For this review, take the finished solid that the model builds, in its own axes (mm). A direction names the side the tool comes from. Give positions to 0.01 mm unless a question says otherwise; leave off trailing zeros. Write each loop counter-clockwise with the first axis right and the second up, starting at its lowest first coordinate (ties: lowest second). Pieces come first, ordered by that corner, then holes. Notation, with made-up numbers: (30, -33) -> (52, -33) arc R8 cw to (52, -28) -> close; hole circle Ø6 at (40.5, 43.5). An arc over 180 degrees is marked (long way). Return JSON: item names as keys, results as strings.
from build123d import *

# Parameters (mm, degrees)
BOSS_EXTRUDE1_DEPTH  = 19.05
CUT_EXTRUDE1_DEPTH   = 23.803574111
SKETCH2_4_W          = 12.954
SKETCH2_4_H          = 1.7018
CUT_EXTRUDE2_DEPTH   = 18.25625
SKETCH6_W            = 0.608326788
SKETCH6_H            = 1.5875
SKETCH8_W            = 2.576826788
SKETCH8_H            = 1.5875
SKETCH9_W            = 12.954
SKETCH9_H            = 5.08
SKETCH9_H_2          = 2.159
CUT_EXTRUDE3_DEPTH   = 6.35
BOSS_EXTRUDE2_DEPTH  = 2.54
SKETCH11_W           = 1.905
SKETCH11_H           = 0.127
BOSS_EXTRUDE3_DEPTH  = 0.254
FILLET1_R            = 0.508
FILLET2_R            = 0.0635
BOSS_EXTRUDE4_DEPTH  = 1.27
BOSS_EXTRUDE5_DEPTH  = 1.905
FILLET1_OF_MIRROR1_R = 0.508


with BuildPart() as part:
    # Sketch1 → Boss-Extrude1 (new body)
    with BuildSketch(Plane(origin=(0, 0, 0), x_dir=(1, 0, 0), z_dir=(0, 1, 0))):
        with BuildLine():
            Line((-0.79375, 9.109483901), (-0.79375, 8.535673212))
            ThreePointArc((-0.79375, 8.535673212), (-7.424002774, 4.28625), (-7.78898484, -3.580428942))
            Line((-7.78898484, -3.580428942), (-8.285919473, -3.867334286))
            ThreePointArc((-8.285919473, -3.867334286), (-7.918936292, -4.572), (-7.492169473, -5.242149615))
            Line((-7.492169473, -5.242149615), (-6.99523484, -4.95524427))
            ThreePointArc((-6.99523484, -4.95524427), (0, -8.5725), (6.99523484, -4.95524427))
            Line((6.99523484, -4.95524427), (7.492169473, -5.242149615))
            ThreePointArc((7.492169473, -5.242149615), (7.918936292, -4.572), (8.285919473, -3.867334286))
            Line((8.285919473, -3.867334286), (7.78898484, -3.580428942))
            ThreePointArc((7.78898484, -3.580428942), (7.424002774, 4.28625), (0.79375, 8.535673212))
            Line((0.79375, 8.535673212), (0.79375, 9.109483901))
            ThreePointArc((0.79375, 9.109483901), (0, 9.144), (-0.79375, 9.109483901))
        make_face()
    extrude(amount=BOSS_EXTRUDE1_DEPTH)

    # Sketch2 → Cut-Extrude1 (cut, through all)
    with BuildSketch(Plane(origin=(0, 19.05, 0), x_dir=(1, 0, 0), z_dir=(0, 1, 0))):
        with BuildLine():
            Line((-4.543615348, 4.303093955), (-3.175, 2.4638))
            Line((-3.175, 2.4638), (3.175, 2.4638))
            Line((3.175, 2.4638), (4.543615348, 4.303093955))
            ThreePointArc((4.543615348, 4.303093955), (4.598203733, 4.928342625), (4.064, 5.2578))
            Line((4.064, 5.2578), (-4.064, 5.2578))
            ThreePointArc((-4.064, 5.2578), (-4.598203733, 4.928342625), (-4.543615348, 4.303093955))
        make_face()
    extrude(amount=-CUT_EXTRUDE1_DEPTH, mode=Mode.SUBTRACT)

    # Sketch2_4 → Cut-Extrude2 (cut)
    with BuildSketch(Plane(origin=(0, 19.05, 0), x_dir=(1, 0, 0), z_dir=(0, 1, 0))):
        with Locations((0, 1.6129)):
            Rectangle(SKETCH2_4_W, SKETCH2_4_H)
    extrude(amount=-CUT_EXTRUDE2_DEPTH, mode=Mode.SUBTRACT)

    # Sketch6 → Cut-Revolve2 (revolve, cut)
    with BuildSketch(Plane(origin=(0, 0, 0), x_dir=(0, 0, -1), z_dir=(1, 0, 0)), mode=Mode.PRIVATE) as cut_revolve2_sk:
        with Locations((8.839836606, 0.79375)):
            Rectangle(SKETCH6_W, SKETCH6_H)
    revolve(cut_revolve2_sk.sketch.rotate(Axis((0, 19.730213777, 0), (0, -1, 0)), 180), axis=Axis((0, 19.730213777, 0), (0, -1, 0)), mode=Mode.SUBTRACT)

    # Sketch8 → Revolve2 (revolve)
    with BuildSketch(Plane(origin=(0, 0, 0), x_dir=(0, 0, -1), z_dir=(1, 0, 0)), mode=Mode.PRIVATE) as revolve2_sk:
        with Locations((9.824086606, 0.79375)):
            Rectangle(SKETCH8_W, SKETCH8_H)
    revolve(revolve2_sk.sketch.rotate(Axis((0, 4.48386458, 0), (0, -1, 0)), 180), axis=Axis((0, 4.48386458, 0), (0, -1, 0)))

    # Sketch9 → Cut-Extrude3 (cut)
    with BuildSketch(Plane(origin=(0, 19.05, 0), x_dir=(1, 0, 0), z_dir=(0, 1, 0))):
        with Locations((0, -1.778)):
            Rectangle(SKETCH9_W, SKETCH9_H)
        with Locations((0, 3.5433)):
            Rectangle(SKETCH9_W, SKETCH9_H_2)
    extrude(amount=-CUT_EXTRUDE3_DEPTH, mode=Mode.SUBTRACT)

    # Sketch10 → Boss-Extrude2 (add)
    with BuildSketch(Plane(origin=(0, 12.7, 0), x_dir=(1, 0, 0), z_dir=(0, 1, 0))):
        Polygon((-3.175, 2.4638), (-4.025504259, 3.6068), (-5.08, 3.6068), (-5.08, 2.4638), align=None)
    boss_extrude2 = extrude(amount=BOSS_EXTRUDE2_DEPTH)

    # Sketch11 → Boss-Extrude3 (add)
    with BuildSketch(Plane.XY.offset(-2.4638)):
        with Locations((-4.1275, 15.1765)):
            Rectangle(SKETCH11_W, SKETCH11_H)
    boss_extrude3 = extrude(amount=BOSS_EXTRUDE3_DEPTH)

    # Fillet1
    fillet1_edges = [part.edges().sort_by_distance(p)[0] for p in [
        (-4.55275213, 12.7, -3.6068),
    ]]
    fillet(fillet1_edges, radius=FILLET1_R)

    # Fillet2
    fillet2_edges = [part.edges().sort_by_distance(p)[0] for p in [
        (-4.1275, 15.113, -2.4638),
    ]]
    fillet(fillet2_edges, radius=FILLET2_R)

    # Sketch12 → Boss-Extrude4 (add)
    with BuildSketch(Plane(origin=(0, 15.24, 0), x_dir=(1, 0, 0), z_dir=(0, 1, 0))):
        Polygon((-3.175, 2.2098), (-3.175, 2.4638), (-4.025504259, 3.6068), (-5.08, 3.6068), (-5.08, 2.2098), align=None)
    boss_extrude4 = extrude(amount=BOSS_EXTRUDE4_DEPTH)

    # Sketch13 → Boss-Extrude5 (add)
    with BuildSketch(Plane(origin=(-3.175, 0, 0), x_dir=(0, 0, -1), z_dir=(1, 0, 0))):
        Polygon((2.2098, 15.113), (1.403241674, 16.51), (2.2098, 16.51), align=None)
    boss_extrude5 = extrude(amount=-BOSS_EXTRUDE5_DEPTH)

    # Mirror1: Boss-Extrude2, Boss-Extrude3, Boss-Extrude4, Boss-Extrude5 across plane
    add(boss_extrude2.mirror(Plane(origin=(0, 0, 0), x_dir=(0, 0, 1), z_dir=(1, 0, 0))))
    add(boss_extrude3.mirror(Plane(origin=(0, 0, 0), x_dir=(0, 0, 1), z_dir=(1, 0, 0))))
    add(boss_extrude4.mirror(Plane(origin=(0, 0, 0), x_dir=(0, 0, 1), z_dir=(1, 0, 0))))
    add(boss_extrude5.mirror(Plane(origin=(0, 0, 0), x_dir=(0, 0, 1), z_dir=(1, 0, 0))))

    # Fillet1 of Mirror1
    fillet1_of_mirror1_edges = [part.edges().sort_by_distance(p)[0] for p in [
        (4.55275213, 12.7, -3.6068),
    ]]
    fillet(fillet1_of_mirror1_edges, radius=FILLET1_OF_MIRROR1_R)


solid = part.part
1. For pin 1 (1.7 mm diameter, centred on x = 5, y = 5, fed in from +Z); pin 2 (3 mm diameter, centred on y = 15, z = -3, fed in from -X); pin 3 (3 mm diameter, centred on x = 1.5, y = 17, fed in from -Z), all flat-tipped, find the tip position at first contact; note any pin that passes through.
Results found:
{"pin 1": "stops at z = 7.5", "pin 2": "stops at x = -8.44", "pin 3": "stops at z = -9.14"}
2. Add section B-B, the plane y = 5.75. State the section outline as (x, z) points (1 decimal).
Results found:
{"outline": "(-8.3, 3.9) -> (-7.8, 3.6) arc R8.6 ccw to (-0.8, -8.5) -> (-0.8, -9.1) arc R9.1 ccw to (0.8, -9.1) -> (0.8, -8.5) arc R8.6 ccw to (7.8, 3.6) -> (8.3, 3.9) arc R9.1 ccw to (7.5, 5.2) -> (7, 5) arc R8.6 ccw to (-7, 5) -> (-7.5, 5.2) arc R9.1 ccw to start; hole (-6.5, -2.5) -> (-3.2, -2.5) -> (-4.5, -4.3) arc R0.6 ccw to (-4.1, -5.3) -> (4.1, -5.3) arc R0.6 ccw to (4.5, -4.3) -> (3.2, -2.5) -> (6.5, -2.5) -> (6.5, -0.8) -> (-6.5, -0.8) -> close"}
3. To check wall thickness, follow probe 1 along Z at (x, y) = (5, 14.5); probe 2 along Y at (x, z) = (-8.25, -5.75); probe 3 along X at (y, z) = (4.25, -2.5). State the ranges of each line that lie inside material, in increasing order.
Results found:
{"probe 1": "z = -6.96 to -4.62, -3.61 to -2.46, 4.32 to 6.96", "probe 2": "y = 0 to 1.59", "probe 3": "x = -8.2 to -3.2, 3.2 to 8.2"}
4. The part is to be moulded in two halves that separate along Z. For faces 4 (the flat face through (0, 0, 0)), 5 (the cylindrical face through (-7.5, 0.8, -8.2)), 6 (the flat face through (3.175, 16, -2)), say which applies: +Z half, -Z half, draft (parallel to the pull), parting line (faces both ways), or undercut.
Results found:
{"face 4": "draft", "face 5": "parting line", "face 6": "undercut"}
5. Add section C-C, the plane z = 0. State the section outline as (x, y) points, plus the area to 3 significant figures.
Results found:
{"outline": "(-11.11, 0) -> (11.11, 0) -> (11.11, 1.59) -> (8.57, 1.59) -> (8.57, 19.05) -> (6.48, 19.05) -> (6.48, 12.7) -> (-6.48, 12.7) -> (-6.48, 19.05) -> (-8.57, 19.05) -> (-8.57, 1.59) -> (-11.11, 1.59) -> close", "area": "252 mm²"}
6. For faces 1 (the flat face through (0, 0.794, -2)), 2 (the flat face through (6, 16, -4.623)), 3 (the cylindrical face through (-7.366, 10.197, -4.385)), list the 3-axis set-ups (+Z, -Z, +X, -X, +Y, -Y) from which the entire face can be reached by the end or side of a thin tool; tool diameter is ignored.
Results found:
{"face 1": "none", "face 2": "+Y", "face 3": "-X, +Y"}
7. Add section D-D, the plane x = -5.5. State the section outline as (y, z) points, plus the area to 3 significant figures.
Results found:
{"outline": "(0, -9.66) -> (1.59, -9.66) -> (1.59, -6.58) -> (19.05, -6.58) -> (19.05, -4.62) -> (12.7, -4.62) -> (12.7, -2.46) -> (0.79, -2.46) -> (0.79, -0.76) -> (12.7, -0.76) -> (12.7, 4.32) -> (19.05, 4.32) -> (19.05, 6.58) -> (1.59, 6.58) -> (1.59, 9.66) -> (0, 9.66) -> close", "area": "183 mm²"}
8. Add section A-A, the plane x = 0. State the section outline as (y, z) points, plus the area to 3 significant figures.
Results found:
{"outline": "(0, -11.11) -> (1.59, -11.11) -> (1.59, -9.14) -> (19.05, -9.14) -> (19.05, -5.26) -> (0, -5.26) -> close; (0, -2.46) -> (0.79, -2.46) -> (0.79, -0.76) -> (12.7, -0.76) -> (12.7, 4.32) -> (19.05, 4.32) -> (19.05, 8.57) -> (1.59, 8.57) -> (1.59, 11.11) -> (0, 11.11) -> close", "area": "228 mm²"}
